Part model, mm, in its own coordinate system. Round coordinates to 2 decimals unless told otherwise and drop trailing zeros. Write each loop counter-clockwise with the first axis right and the second up, starting at its lowest first coordinate (ties: lowest second). Pieces come first, ordered by that corner, then holes. Notation, with made-up numbers: (-8, 82.5) -> (-1, 82.5) arc R32 cw to (-1, 116.5) -> close; hole circle Ø3 at (38, 70). An arc over 180 degrees is marked (long way). Use CSV: the item, a comma, the result in double quotes. Start each with the question number.
(1) Probe line 1 (X direction, y = 2.15, z = -76). List the from-to ranges inside material, lowest first. Write a range as [from, to].
(2) Drop flat-ended pins along their axis: pin 1 (1.5 mm diameter, centred on x = 3.5, y = 2, fed in from +Z); pin 2 (1 mm diameter, centred on x = 0, z = 20.5, fed in from -Y); pin 3 (1.5 mm diameter, centred on x = -28.5, y = 1, fed in from -Z); pin 4 (0.9 mm diameter, centred on x = 3, y = 1.5, fed in from -Z). Give the stop position or say it passes through.
(3) Saw through at A-A (y = 0.5). Give the cut face in (x, z), plus the area to 3 significant figures.
(4) Saw through at B-B (z = 36). Give the cut face in (x, y), plus the area to 3 significant figures.
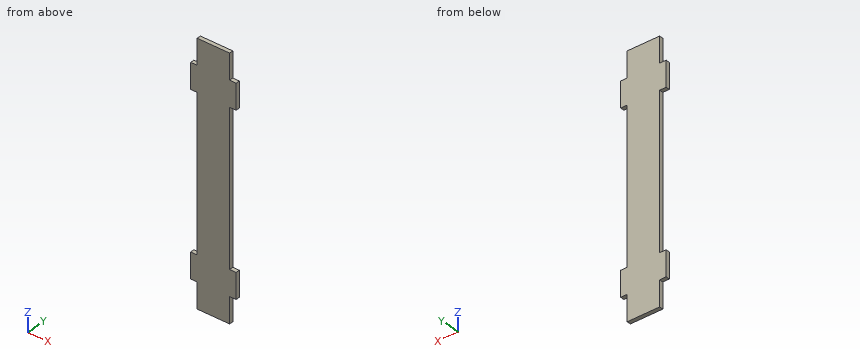
```python
from build123d import *

# Parameters (mm, degrees)
F0_W     = 5
F0_H     = 20
F1_DEPTH = 3


with BuildPart() as f1:
    # F0 (on Front) → F1 (new body)
    with BuildSketch(Plane.XZ):
        Polygon((0, 107.721728), (-25, 107.721728), (-25, 87.721728), (-25, 67.721728), (-25, -52.278272), (-25, -72.278272), (-25, -92.278272), (0, -92.278272), (0, -72.278272), (0, -72.036713), (0, -52.036713), (0, 67.721728), (0, 87.721728), align=None)
        with Locations((2.5, 77.721728)):
            Rectangle(F0_W, F0_H)
        with Locations((-27.5, 77.721728)):
            Rectangle(F0_W, F0_H)
        Polygon((3, -52.036713), (0, -52.036713), (0, -72.036713), (5, -72.036713), (5, -52.036713), align=None)
        Polygon((-25, -72.278272), (-25, -52.278272), (-28, -52.278272), (-30, -52.278272), (-30, -72.278272), (-28, -72.278272), align=None)
    extrude(amount=-F1_DEPTH)


solid = f1.part
```
Answers:
1,line 1,"x = [-25, 0]"
2,pin 1,"stops at z = 87.72"
2,pin 2,"stops at y = 0"
2,pin 3,"stops at z = -72.28"
2,pin 4,"stops at z = -72.04"
3,outline,"(-30, -72.28) -> (-25, -72.28) -> (-25, -92.28) -> (0, -92.28) -> (0, -72.04) -> (5, -72.04) -> (5, -52.04) -> (0, -52.04) -> (0, 67.72) -> (5, 67.72) -> (5, 87.72) -> (0, 87.72) -> (0, 107.72) -> (-25, 107.72) -> (-25, 87.72) -> (-30, 87.72) -> (-30, 67.72) -> (-25, 67.72) -> (-25, -52.28) -> (-30, -52.28) -> close"
3,area,"5,400 mm²"
4,outline,"(-25, 0) -> (0, 0) -> (0, 3) -> (-25, 3) -> close"
4,area,"75.0 mm²"
